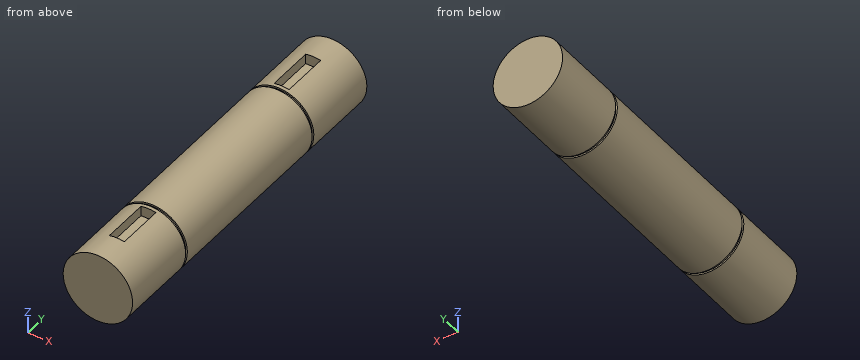
```python
from build123d import *

# Parameters (mm, degrees)
SKETCH1_R           = 32.5
BOSS_EXTRUDE1_DEPTH = 326
SKETCH2_R           = 53.453114337
SKETCH2_R_2         = 31
CUT_EXTRUDE1_DEPTH  = 2.42
CUT_EXTRUDE2_START  = 2.42
SKETCH3_R           = 95.953037666
SKETCH3_R_2         = 31
CUT_EXTRUDE2_DEPTH  = 2.42
SKETCH5_W           = 14
SKETCH5_H           = 44
CUT_EXTRUDE3_DEPTH  = 10


with BuildPart() as part:
    # Sketch1 → Boss-Extrude1 (new body)
    with BuildSketch(Plane(origin=(0, 0, 0), x_dir=(1, 0, 0), z_dir=(0, 1, 0))):
        with Locations(Location((0, 0, 0), (0, 0, 270))):
            Circle(SKETCH1_R)
    extrude(amount=BOSS_EXTRUDE1_DEPTH)

    # Sketch2 → Cut-Extrude1 (cut)
    with BuildSketch(Plane(origin=(0, 73.8, 0), x_dir=(1, 0, 0), z_dir=(0, 1, 0))):
        Circle(SKETCH2_R)
        with Locations(Location((0, 0, 0), (0, 0, 90))):
            Circle(SKETCH2_R_2, mode=Mode.SUBTRACT)
    extrude(amount=CUT_EXTRUDE1_DEPTH, mode=Mode.SUBTRACT)

    # Sketch3 → Cut-Extrude2 (cut)
    with BuildSketch(Plane(origin=(0, 252.2, 0), x_dir=(-1, 0, 0), z_dir=(0, -1, 0)).offset(CUT_EXTRUDE2_START)):
        Circle(SKETCH3_R)
        with Locations(Location((0, 0, 0), (0, 0, 90))):
            Circle(SKETCH3_R_2, mode=Mode.SUBTRACT)
    extrude(amount=-CUT_EXTRUDE2_DEPTH, mode=Mode.SUBTRACT)

    # Sketch5 → Cut-Extrude3 (cut)
    with BuildSketch(Plane.XY.offset(32.5)):
        with Locations((0, 277.6)):
            Rectangle(SKETCH5_W, SKETCH5_H)
        with Locations((0, 48.4)):
            Rectangle(SKETCH5_W, SKETCH5_H)
    extrude(amount=-CUT_EXTRUDE3_DEPTH, mode=Mode.SUBTRACT)


solid = part.part
```
Part model, mm, in its own coordinate system. Round coordinates to 2 decimals unless told otherwise and drop trailing zeros. Loops run counter-clockwise (first coordinate to the right, second up) from the corner with the lowest first, then second, coordinate; pieces in that order, holes last. Notation, with made-up numbers: (-26.5, 19.5) -> (29.5, 19.5) arc R23 ccw to (29.5, 50.5) -> close; hole circle Ø3 at (16.25, 51). An arc over 180 degrees is marked (long way). Use one line per item in the form item = value. Start each with the question number.
Item 1: Drop flat-ended pins along their axis: pin 1 Ø8 at (x, z) = (-2.5, 25) entering from -Y; pin 2 Ø11 at (x, y) = (-2.5, 42) entering from +Z; pin 3 Ø2 at (x, y) = (-9.5, 223) entering from +Z; pin 4 Ø7 at (x, y) = (-1, 287.5) entering from +Z. Give the stop position or say it passes through.
Item 2: Band-saw the part on D-D (x = 0). List the corners of the cut face in (y, z), plus the area to 3 significant figures.
Item 3: Band-saw the part on C-C (y = 219.5). List the corners of the cut face in (x, z).
Item 4: Drill centre lines: line 1 along Z through (x, y) = (1.5, 229.5); line 2 along X through (y, z) = (280.5, 0); line 3 along X through (y, z) = (229, 9). Where is each one in solid material? Low to high.
Item 5: Band-saw the part on A-A (x = -24). List the corners of the cut face in (y, z), plus the area to 3 significant figures.
Item 6: Band-saw the part on B-B (z = 13.5). List the corners of the cut face in (x, y).
Data:
q1.pin_1 = 0
q1.pin_2 = 31.74
q1.pin_3 = 31.37
q1.pin_4 = 22.5
q2.outline = (0, -32.5) -> (73.8, -32.5) -> (73.8, -31) -> (76.22, -31) -> (76.22, -32.5) -> (249.78, -32.5) -> (249.78, -31) -> (252.2, -31) -> (252.2, -32.5) -> (326, -32.5) -> (326, 32.5) -> (299.6, 32.5) -> (299.6, 22.5) -> (255.6, 22.5) -> (255.6, 32.5) -> (252.2, 32.5) -> (252.2, 31) -> (249.78, 31) -> (249.78, 32.5) -> (76.22, 32.5) -> (76.22, 31) -> (73.8, 31) -> (73.8, 32.5) -> (70.4, 32.5) -> (70.4, 22.5) -> (26.4, 22.5) -> (26.4, 32.5) -> (0, 32.5) -> close
q2.area = 20,300 mm^2
q3.outline = circle Ø65 at (0, 0)
q4.line_1 = -32.47 to 32.47
q4.line_2 = -32.5 to 32.5
q4.line_3 = -31.23 to 31.23
q5.outline = (0, -21.91) -> (73.8, -21.91) -> (73.8, -19.62) -> (76.22, -19.62) -> (76.22, -21.91) -> (249.78, -21.91) -> (249.78, -19.62) -> (252.2, -19.62) -> (252.2, -21.91) -> (326, -21.91) -> (326, 21.91) -> (252.2, 21.91) -> (252.2, 19.62) -> (249.78, 19.62) -> (249.78, 21.91) -> (76.22, 21.91) -> (76.22, 19.62) -> (73.8, 19.62) -> (73.8, 21.91) -> (0, 21.91) -> close
q5.area = 14,300 mm^2
q6.outline = (-29.56, 0) -> (29.56, 0) -> (29.56, 73.8) -> (27.91, 73.8) -> (27.91, 76.22) -> (29.56, 76.22) -> (29.56, 249.78) -> (27.91, 249.78) -> (27.91, 252.2) -> (29.56, 252.2) -> (29.56, 326) -> (-29.56, 326) -> (-29.56, 252.2) -> (-27.91, 252.2) -> (-27.91, 249.78) -> (-29.56, 249.78) -> (-29.56, 76.22) -> (-27.91, 76.22) -> (-27.91, 73.8) -> (-29.56, 73.8) -> close
